from build123d import *

# Parameters (mm, degrees)
F0_W      = 43.5
F0_H      = 20
F1_DEPTH  = 21
F3_R      = 3
F4_DEPTH  = 20.001
F2_R      = 2
F5_DEPTH  = 16.5
F6_W      = 22
F6_H      = 14.5
F6_R      = 3
F7_DEPTH  = 14
F11_DEPTH = 21.001
F12_W     = 9.75
F12_H     = 3
F12_W_2   = 23.5
F12_H_2   = 2
F13_DEPTH = 21.001
F14_W     = 11
F14_H     = 3
F15_DEPTH = 43.501


with BuildPart() as f1:
    # F0 (on Front) → F1 (new body)
    with BuildSketch(Plane.XZ):
        with Locations((21.75, 10)):
            Rectangle(F0_W, F0_H)
    extrude(amount=F1_DEPTH)

    # F3 (on face) → F4 (cut, through all)
    with BuildSketch(Plane.XY.offset(20)):
        with Locations((35.5, -10.5)):
            Circle(F3_R)
    extrude(amount=-F4_DEPTH, mode=Mode.SUBTRACT)

    # F2 (on face) → F5 (cut)
    with BuildSketch(Plane.XY.offset(20)):
        with Locations((11, -10.5)):
            Circle(F2_R)
    extrude(amount=-F5_DEPTH, mode=Mode.SUBTRACT)

    # F6 (on face) → F7 (cut)
    with BuildSketch(Plane.XY.offset(20)):
        with Locations((32.5, -10.75)):
            Rectangle(F6_W, F6_H)
        with Locations((35.5, -10.5)):
            Circle(F6_R, mode=Mode.SUBTRACT)
    extrude(amount=-F7_DEPTH, mode=Mode.SUBTRACT)

    # F10 (on face) → F11 (cut, through all)
    with BuildSketch(Plane.XZ.offset(21)):
        Polygon((43.5, 6), (43.5, 20), (21.75, 20), (21.75, 14.5), align=None)
    extrude(amount=-F11_DEPTH, mode=Mode.SUBTRACT)

    # F12 (on face) → F13 (cut, through all)
    with BuildSketch(Plane.XZ.offset(21)):
        with Locations((10.875, 16)):
            Rectangle(F12_W, F12_H)
        Polygon((18.25, 20), (3.5, 20), (3.5, 17.5), (6, 17.5), (15.75, 17.5), (18.25, 17.5), align=None)
        with Locations((17.25, 1)):
            Rectangle(F12_W_2, F12_H_2)
    extrude(amount=-F13_DEPTH, mode=Mode.SUBTRACT)

    # F14 (on face) → F15 (cut, through all)
    with BuildSketch(Plane(origin=(0, 0, 0), x_dir=(0, -1, 0), z_dir=(-1, 0, 0))):
        Polygon((18.5, 20), (2.5, 20), (2.5, 17.5), (5, 17.5), (16, 17.5), (18.5, 17.5), align=None)
        with Locations((10.5, 16)):
            Rectangle(F14_W, F14_H)
    extrude(amount=-F15_DEPTH, mode=Mode.SUBTRACT)


solid = f1.part
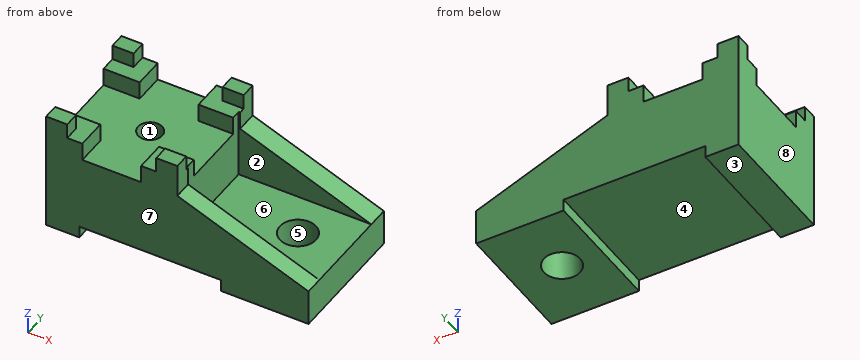
Here's how the part is built. I have some questions about the finished solid (model axes, mm). Face numbers are marked on the shaded views. A direction names the side the tool comes from. Coordinates: 2 decimals unless noted, no trailing zeros. Write each loop counter-clockwise with the first axis right and the second up, starting at its lowest first coordinate (ties: lowest second). Pieces come first, ordered by that corner, then holes. Notation, with made-up numbers: (55.5, 86.25) - (84.5, 86.25) arc R35 ccw to (84.5, 118.25) - close; hole circle Ø2 at (74.5, 88). An arc over 180 degrees is marked (long way). Use one line per item in the form item = value.
1) Suppose I cut it at B-B, the plane x = 33. Write out the boundary of the cut face in (y, z), plus the area to 3 significant figures.
Solved:
outline = (-21, 0) - (-12.16, 0) - (-12.16, 6) - (-18, 6) - (-18, 10.1) - (-21, 10.1) - close; (-8.84, 0) - (0, 0) - (0, 10.1) - (-3.5, 10.1) - (-3.5, 6) - (-8.84, 6) - close
area = 133 mm2
2) I need wall thicknesses on line 1 (Y direction, x = 11, z = 8); line 2 (Y direction, x = 28.5, z = 7); line 3 (X direction, y = -18.5, z = 1.75). Which ranges of each line are inside material? Lowest first, please.
Solved:
line_1 = -21 to -12.5, -8.5 to 0
line_2 = -21 to -18, -3.5 to 0
line_3 = 0 to 5.5, 29 to 43.5
3) Suppose I cut it at A-A, the plane y = -10.5. Write out the boundary of the cut face in (x, z).
Solved:
outline = (0, 0) - (5.5, 0) - (5.5, 2) - (29, 2) - (29, 0) - (32.5, 0) - (32.5, 6) - (21.5, 6) - (21.5, 14.5) - (13, 14.5) - (13, 3.5) - (9, 3.5) - (9, 14.5) - (0, 14.5) - close; (38.5, 0) - (43.5, 0) - (43.5, 6) - (38.5, 6) - close
4) Suppose I cut it at D-D, the plane x = 11. Write out the boundary of the cut face in (y, z), plus the area to 4 significant figures.
Solved:
outline = (-21, 2) - (0, 2) - (0, 14.5) - (-8.5, 14.5) - (-8.5, 3.5) - (-12.5, 3.5) - (-12.5, 14.5) - (-21, 14.5) - close
area = 218.5 mm2
5) I'm going to push flat-ended pins straight in: P1, Ø1.2, axis at y = -1, z = 18.5, coming from the -X side; P2, Ø0.9, axis at y = -1.5, z = 16, coming from the +X side; P3, Ø6, axis at x = 30, z = 15.5, coming from the +Y side; P4, Ø6.5, axis at x = 14.5, y = -15, coming from the -Z side. Where does each tip first touch, or does it pass through?
Solved:
P1 = 0
P2 = 21.75
P3 = through
P4 = 2
6) On a 3-axis mill with a long thin cutter (end or side, diameter ignored), from which of +Z, -Z, +X, -X, +Y, -Y can I reach the whole of each face in a straight line? I mean the marked faces 1, 2, 3 and 4. Say none if no direction works.
Solved:
face_1 = +Z
face_2 = +Z, +X
face_3 = -Z, +X, -X, +Y, -Y
face_4 = -Z, +Y, -Y
7) Thinking about a two-plate mould opening in Y: for the marked faces 5, 6, 7 and 8, which applies, released by +Y, released by -Y, zero draft, split by the parting line, or undercut?
Solved:
face_5 = undercut
face_6 = undercut
face_7 = released by -Y
face_8 = zero draft
8) Suppose I cut it at C-C, the plane z = 6.75. Write out the boundary of the cut face in (x, y).
Solved:
outline = (0, -21) - (41.58, -21) - (41.58, -18) - (21.5, -18) - (21.5, -3.5) - (41.58, -3.5) - (41.58, 0) - (0, 0) - close; hole circle Ø4 at (11, -10.5)
